Part print with two shaded views. Sizes in mm from the minimum x, y, z corner. Round coordinates to 2 decimals unless told otherwise and drop trailing zeros. Order: outer loops, then holes, each group sorted by start corner. A loop starts at its lowest first (then second) coordinate and runs counter-clockwise, first axis right, second up. Notation, with made-up numbers: (25, 49.25) -> (48, 49.25) arc R11 ccw to (48, 70.25) -> close; hole circle Ø6 at (33, -36.75). An arc over 180 degrees is marked (long way). Put each result on its own line as item: value. Start each with the question number.
Q1. Cut at D-D, the plane x = 46. List the corners of the cut face in (y, z), and give its area (3 significant figures).
Q2. Cut at B-B, the plane z = 3.35. State how many separate pieces and enclosed holes the cut face has, and give its area (3 significant figures).
Q3. Flat gauge pins, fed straight in: P1, Ø2.5, axis at x = 76, y = 3.5, coming from the -Z side; P2, Ø1, axis at x = 88.5, y = 7, coming from the -Z side. Where does each tip first touch, or does it go through?
Q4. Cut at C-C, the plane y = 10.5. List the corners of the cut face in (x, z).
Q5. Cut at A-A, the plane x = 4. List the corners of the cut face in (y, z), and give its area (3 significant figures).
Q6. Probe L1, parallel to X at y = 3.5, z = 1.6; L2, parallel to X at y = 12, z = 2.95; L3, parallel to Y at x = 90, z = 0.65. List the from-to ranges inside material, lowest first.
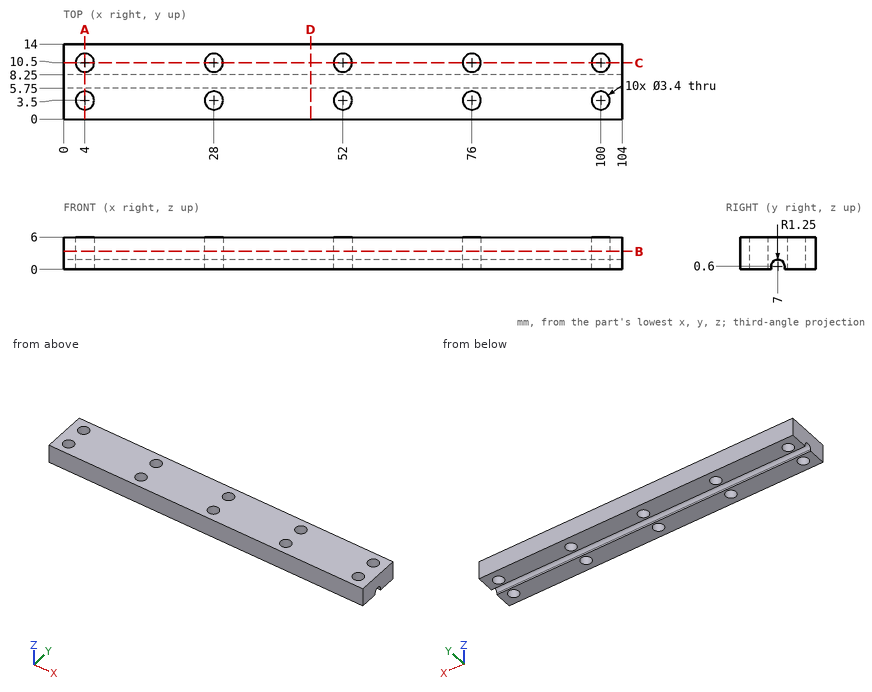
Ans:
1. outline: (0, 0) -> (5.75, 0) -> (5.75, 0.6) arc R1.25 cw to (8.25, 0.6) -> (8.25, 0) -> (14, 0) -> (14, 6) -> (0, 6) -> close
1. area: 80.0 mm^2
2. separate pieces: 1
2. enclosed holes: 10
2. area: 1,370 mm^2
3. P1: passes through
3. P2: stops at z = 1.75
4. outline: (0, 0) -> (2.3, 0) -> (2.3, 6) -> (0, 6) -> close; (5.7, 0) -> (26.3, 0) -> (26.3, 6) -> (5.7, 6) -> close; (29.7, 0) -> (50.3, 0) -> (50.3, 6) -> (29.7, 6) -> close; (53.7, 0) -> (74.3, 0) -> (74.3, 6) -> (53.7, 6) -> close; (77.7, 0) -> (98.3, 0) -> (98.3, 6) -> (77.7, 6) -> close; (101.7, 0) -> (104, 0) -> (104, 6) -> (101.7, 6) -> close
5. outline: (0, 0) -> (1.8, 0) -> (1.8, 6) -> (0, 6) -> close; (5.2, 0) -> (5.75, 0) -> (5.75, 0.6) arc R1.25 cw to (8.25, 0.6) -> (8.25, 0) -> (8.8, 0) -> (8.8, 6) -> (5.2, 6) -> close; (12.2, 0) -> (14, 0) -> (14, 6) -> (12.2, 6) -> close
5. area: 39.2 mm^2
6. L1: x = 0 to 2.3, 5.7 to 26.3, 29.7 to 50.3, 53.7 to 74.3, 77.7 to 98.3, 101.7 to 104
6. L2: x = 0 to 3.2, 4.8 to 27.2, 28.8 to 51.2, 52.8 to 75.2, 76.8 to 99.2, 100.8 to 104
6. L3: y = 0 to 5.75, 8.25 to 14
